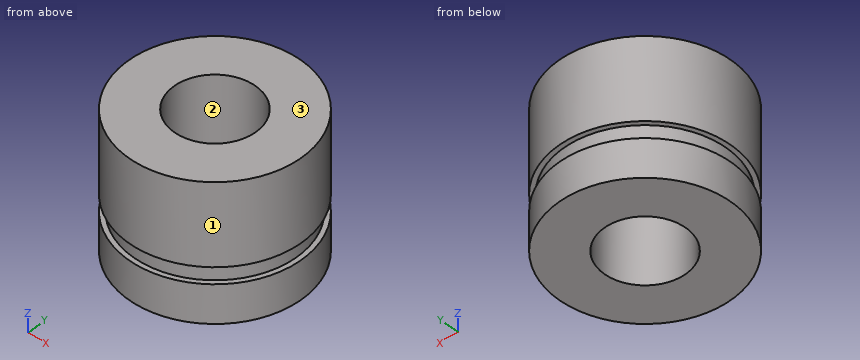
```python
from build123d import *

# Parameters (mm, degrees)
F0_R     = 15.875
F0_R_2   = 7.5
F1_DEPTH = 25
F3_R     = 15.875
F3_R_2   = 15
F4_DEPTH = 3


with BuildPart() as f1:
    # F0 (on Top) → F1 (new body)
    with BuildSketch(Plane.XY):
        Circle(F0_R)
        Circle(F0_R_2, mode=Mode.SUBTRACT)
    extrude(amount=F1_DEPTH)

    # F3 (on offset) → F4 (cut)
    with BuildSketch(Plane.XY.offset(7)):
        Circle(F3_R)
        Circle(F3_R_2, mode=Mode.SUBTRACT)
    extrude(amount=F4_DEPTH, mode=Mode.SUBTRACT)


solid = f1.part
```
Geometry check sheet. Reference: the model listing, model coordinates, mm. Face numbers are marked on the shaded views. Coordinates: 2 decimals unless noted, no trailing zeros. Order: outer loops, then holes, each group sorted by start corner. A loop starts at its lowest first (then second) coordinate and runs counter-clockwise, first axis right, second up. Notation, with made-up numbers: (72.5, 62) - (77.5, 62) arc R12 ccw to (77.5, 72) - close; hole circle Ø6 at (0, -23.5). An arc over 180 degrees is marked (long way). Answer in a Markdown table with one row per item. Add a question column.
1. Section check A-A (y = 0). Enter the section's corners in (x, z) (3 decimals), plus the area to 4 significant figures.
2. Draft check along Y on the marked faces 1, 2 and 3. Enter one of: +Y half, -Y half, draft (parallel to the pull), parting line (faces both ways), or undercut.
3. Gauge pin test, flat ends, axial feed: pin 1 Ø12 at (x, z) = (-9, 2.5) entering from -Y; pin 2 Ø4 at (y, z) = (6.5, 9) entering from -X; pin 3 Ø2 at (y, z) = (8.5, 16) entering from -X. Record the tip position at first contact, or that the pin passes through.
4. Section check C-C (z = 15.25). Enter the section's corners in (x, y) (3 decimals), plus the area to 3 significant figures.
5. Section check D-D (x = -12.5). Enter the section's corners in (y, z), plus the area to 3 significant figures.
6. Material ranges on L1, parallel to Y at x = 0, z = 8.75; L2, parallel to Y at x = 0, z = 10.75 (3 decimals); L3, parallel to X at y = 6, z = 6.75, recorded low to high. Write a range as [from, to].
Data:
| question | item | result |
|---|---|---|
| 1 | outline | (-15.875, 0) - (-7.5, 0) - (-7.5, 25) - (-15.875, 25) - (-15.875, 10) - (-15, 10) - (-15, 7) - (-15.875, 7) - close; (7.5, 0) - (15.875, 0) - (15.875, 7) - (15, 7) - (15, 10) - (15.875, 10) - (15.875, 25) - (7.5, 25) - close |
| 1 | area | 413.5 mm² |
| 2 | face 1 | parting line |
| 2 | face 2 | undercut |
| 2 | face 3 | draft |
| 3 | pin 1 | stops at y = -15.59 |
| 3 | pin 2 | stops at x = -15.14 |
| 3 | pin 3 | stops at x = -13.99 |
| 4 | outline | circle Ø31.75 at (0, 0); hole circle Ø15 at (0, 0) |
| 4 | area | 615 mm² |
| 5 | outline | (-9.79, 0) - (9.79, 0) - (9.79, 7) - (8.29, 7) - (8.29, 10) - (9.79, 10) - (9.79, 25) - (-9.79, 25) - (-9.79, 10) - (-8.29, 10) - (-8.29, 7) - (-9.79, 7) - close |
| 5 | area | 480 mm² |
| 6 | L1 | y = [-15, -7.5], [7.5, 15] |
| 6 | L2 | y = [-15.875, -7.5], [7.5, 15.875] |
| 6 | L3 | x = [-14.7, -4.5], [4.5, 14.7] |
